Input: part model. Units: mm. Frame: model coordinates. Face numbers are marked on the shaded views. A direction names the side the tool comes from. Coordinates: 2 decimals unless noted, no trailing zeros. Write each loop counter-clockwise with the first axis right and the second up, starting at its lowest first coordinate (ties: lowest second). Pieces come first, ordered by that corner, then holes. Notation, with made-up numbers: (0.5, -21) -> (12.5, -21) arc R18 ccw to (12.5, 12) -> close; hole circle Ø7 at (75.25, 88.25). An arc over 180 degrees is marked (long way). One line per question, with ' | ' between items. Start each with the question number.
```python
from build123d import *

# Parameters (mm, degrees)
CROQUIS1_R              = 22.606
SALIENTE_EXTRUIR1_DEPTH = 50.8
CROQUIS2_R              = 12.7
SALIENTE_EXTRUIR2_DEPTH = 56.642
CROQUIS3_R              = 2.54
CORTAR_EXTRUIR1_DEPTH   = 31.242
CROQUIS4_R              = 5.207
CORTAR_EXTRUIR4_DEPTH   = 144.018
SALIENTE_EXTRUIR3_START = -2.286
CROQUIS5_R              = 22.606
SALIENTE_EXTRUIR3_DEPTH = 2.286
C_PULA1_FACE_RADIUS     = 22.606
C_PULA1_HEIGHT          = 2.54


with BuildPart() as part:
    # Croquis1 → Saliente-Extruir1 (new body)
    with BuildSketch(Plane(origin=(0, 0, 0), x_dir=(1, 0, 0), z_dir=(0, 1, 0))):
        with Locations(Location((0, 0, 0), (0, 0, 270))):
            Circle(CROQUIS1_R)
    extrude(amount=SALIENTE_EXTRUIR1_DEPTH)

    # Croquis2 → Saliente-Extruir2 (add)
    with BuildSketch(Plane(origin=(0, 0, 0), x_dir=(1, 0, 0), z_dir=(0, 1, 0))):
        with Locations(Location((0, 0, 0), (0, 0, 270))):
            Circle(CROQUIS2_R)
    extrude(amount=SALIENTE_EXTRUIR2_DEPTH)

    # Croquis3 → Cortar-Extruir1 (cut)
    with BuildSketch(Plane(origin=(0, 0, 0), x_dir=(0, 0, -1), z_dir=(1, 0, 0))):
        with Locations((0, 40.032848535)):
            Circle(CROQUIS3_R)
        with Locations((0, 15.428124721)):
            Circle(CROQUIS3_R)
    extrude(amount=-CORTAR_EXTRUIR1_DEPTH, mode=Mode.SUBTRACT)

    # Croquis4 → Cortar-Extruir4 (cut)
    with BuildSketch(Plane(origin=(0, 0, 0), x_dir=(1, 0, 0), z_dir=(0, 1, 0))):
        with Locations(Location((0, 0, 0), (0, 0, 270))):
            Circle(CROQUIS4_R)
    extrude(amount=CORTAR_EXTRUIR4_DEPTH, mode=Mode.SUBTRACT)

    # Croquis5 → Saliente-Extruir3 (add)
    with BuildSketch(Plane(origin=(0, 0, 0), x_dir=(1, 0, 0), z_dir=(0, 1, 0)).offset(SALIENTE_EXTRUIR3_START)):
        with Locations(Location((0, 0, 0), (0, 0, 270))):
            Circle(CROQUIS5_R)
    extrude(amount=SALIENTE_EXTRUIR3_DEPTH)

    # Cúpula1: a dome of height H over a round flat face of radius A is a cap of a sphere of radius (A * A + H * H) / (2 * H)
    c_pula1_r = (C_PULA1_FACE_RADIUS * C_PULA1_FACE_RADIUS + C_PULA1_HEIGHT * C_PULA1_HEIGHT) / (2 * C_PULA1_HEIGHT)
    c_pula1_base = Plane((0, -2.286, 0), z_dir=(0, -1, 0))
    with Locations(c_pula1_base.offset(C_PULA1_HEIGHT - c_pula1_r)):
        c_pula1_ball = Sphere(c_pula1_r, mode=Mode.PRIVATE)
    add(split(c_pula1_ball, bisect_by=c_pula1_base, keep=Keep.TOP, mode=Mode.PRIVATE))


solid = part.part
```
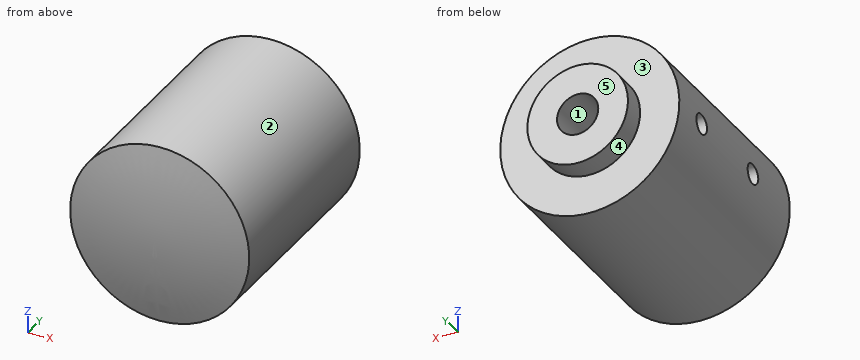
1) Ray query, line 1 (X direction, y = 27, z = 0); line 2 (Y direction, x = -9, z = 0). Return the intervals inside material, ascending.
2) First-contact query: P1, Ø2, axis at x = -11, y = 10, coming from the -Z side; P2, Ø10, axis at y = 4.5, z = -7.5, coming from the +X side; P3, Ø1.5, axis at x = -1, y = 17.5, coming from the +Z side. Flat tips, straight axial feed; report the tip coordinate or a pass-through.
3) Section D-D, the plane z = 8.5. Return loops of the section in (x, y), then the cut area to 3 significant figures.
4) Pull-direction query (X, two-part tool) for the marked faces 1, 2 and 3; classes: released by +X, released by -X, zero draft, split by the parting line, or undercut.
5) Section A-A, the plane z = 0. Return loops of the section in (x, y), then the cut area to 3 significant figures.
6) Access query for the marked faces 4 and 5. Directions: +Z, -Z, +X, -X, +Y, -Y. A direction counts if a zero-diameter tool reaches every point of the face in a straight line with its end or side. Return the directions, or none.
7) Section C-C, the plane y = 1.5. Return loops of the section in (x, z).
8) Section B-B, the plane x = 0. Return loops of the section in (y, z).
Answer block:
1) line 1: x = -22.61 to -5.21, 5.21 to 22.61 | line 2: y = -4.43 to 12.89, 17.97 to 37.49, 42.57 to 56.64
2) P1: stops at z = -20.27 | P2: stops at x = 22.47 | P3: stops at z = 22.6
3) outline: (-20.95, -2.29) arc R101.51 ccw to (20.95, -2.29) -> (20.95, 50.8) -> (9.44, 50.8) -> (9.44, 56.64) -> (-9.44, 56.64) -> (-9.44, 50.8) -> (-20.95, 50.8) -> close | area: 2,400 mm2
4) face 1: undercut | face 2: split by the parting line | face 3: zero draft
5) outline: (-22.61, -2.29) arc R101.87 ccw to (22.61, -2.29) -> (22.61, 50.8) -> (12.7, 50.8) -> (12.7, 56.64) -> (5.21, 56.64) -> (5.21, 0) -> (-5.21, 0) -> (-5.21, 12.89) -> (-22.61, 12.89) -> close; (-22.61, 17.97) -> (-5.21, 17.97) -> (-5.21, 37.49) -> (-22.61, 37.49) -> close; (-22.61, 42.57) -> (-5.21, 42.57) -> (-5.21, 56.64) -> (-12.7, 56.64) -> (-12.7, 50.8) -> (-22.61, 50.8) -> close | area: 1,860 mm2
6) face 4: +Y | face 5: +Z, -Z, +X, -X, +Y
7) outline: circle Ø45.21 at (0, 0); hole circle Ø10.41 at (0, 0)
8) outline: (-2.29, -22.61) -> (50.8, -22.61) -> (50.8, -12.7) -> (56.64, -12.7) -> (56.64, -5.21) -> (0, -5.21) -> (0, 5.21) -> (56.64, 5.21) -> (56.64, 12.7) -> (50.8, 12.7) -> (50.8, 22.61) -> (-2.29, 22.61) arc R101.87 ccw to start
